Read the model definition and answer for the solid it produces. Units are mm, in the model's axes. Face numbers are marked on the shaded views. A direction names the side the tool comes from. Coordinates: 2 decimals unless noted, no trailing zeros. Write each loop counter-clockwise with the first axis right and the second up, starting at its lowest first coordinate (ties: lowest second). Pieces come first, ordered by that corner, then holes.
1) This flat-tipped pin is pushed along its axis until it touches: pin 1 Ø1.6 at (y, z) = (-2.66, -8.3) entering from +X. Where does it stop, or does it pass through?
2) Which of the six approach directions +Z, -Z, +X, -X, +Y, -Y give full straight-line access (tool end or side, diameter ignored) to the marked faces 5 and 6?
3) The part is cut by section A-A (y = -12). Determine the outline of the cut face in (x, z), then the cut area to 4 significant figures.
4) Determine the mould class of the marked faces 1, 2, 3 and 4 for opening direction X: +X half, -X half, draft (parallel to the pull), parting line (faces both ways), or undercut.
5) Find the intervals of material crossed by line 1 (X direction, y = -0.25, z = -15); line 2 (X direction, y = 3.5, z = 2.5); line 3 (Z direction, x = -4.5, y = -1), in increasing order.
6) The part is cut by section B-B (x = 20). Determine the outline of the cut face in (y, z), then the cut area to 3 significant figures.
from build123d import *

# Parameters (mm, degrees)
BOSS_EXTRUDE1_DEPTH = 5
SKETCH4_W           = 5
SKETCH4_H           = 30
BOSS_EXTRUDE4_DEPTH = 35
SKETCH5_R           = 3
CUT_EXTRUDE2_DEPTH  = 40
CUT_EXTRUDE3_DEPTH  = 10
SKETCH7_R           = 1
SKETCH7_R_2         = 1.000000019
CUT_EXTRUDE4_DEPTH  = 10
FILLET2_R           = 3
FILLET3_R           = 3
FILLET5_R           = 3
FILLET6_R           = 3
CUT_EXTRUDE5_DEPTH  = 5


with BuildPart() as part:
    # Sketch1 → Boss-Extrude1 (new body)
    with BuildSketch(Plane.XY):
        with BuildLine():
            Line((5, 0), (36.35, 0))
            Line((36.35, 0), (36.35, 15))
            Line((36.35, 15), (-36.35, 15))
            Line((-36.35, 15), (-36.35, 0))
            Line((-36.35, 0), (-5, 0))
            ThreePointArc((-5, 0), (0, 5), (5, 0))
        make_face()
        with BuildLine():
            ThreePointArc((-5, 0), (0, -5), (5, 0))
            Line((5, 0), (0, 0))
            Line((0, 0), (-5, 0))
        make_face()
        with BuildLine():
            Line((0, 0), (5, 0))
            ThreePointArc((5, 0), (0, 5), (-5, 0))
            Line((-5, 0), (0, 0))
        make_face()
        with BuildLine():
            Line((-36.35, -15), (36.35, -15))
            Line((36.35, -15), (36.35, 0))
            Line((36.35, 0), (5, 0))
            ThreePointArc((5, 0), (0, -5), (-5, 0))
            Line((-5, 0), (-36.35, 0))
            Line((-36.35, 0), (-36.35, -15))
        make_face()
    extrude(amount=BOSS_EXTRUDE1_DEPTH)

    # Sketch4 → Boss-Extrude4 (add)
    with BuildSketch(Plane(origin=(0, 0, 0), x_dir=(-1, 0, 0), z_dir=(0, 0, -1))):
        with Locations((-33.85, 0)):
            Rectangle(SKETCH4_W, SKETCH4_H)
    boss_extrude4 = extrude(amount=BOSS_EXTRUDE4_DEPTH)

    # Sketch5 → Cut-Extrude2 (cut)
    with BuildSketch(Plane(origin=(36.35, 0, 0), x_dir=(0, 0, -1), z_dir=(1, 0, 0))):
        with Locations(Location((20, 0, 0), (0, 0, 90))):
            Circle(SKETCH5_R)
    cut_extrude2 = extrude(amount=-CUT_EXTRUDE2_DEPTH, mode=Mode.SUBTRACT)

    # Sketch6 → Cut-Extrude3 (cut)
    with BuildSketch(Plane.ZY.offset(-31.35)):
        with BuildLine():
            ThreePointArc((-35, 0), (-30.606601718, 10.606601718), (-20, 15))
            Line((-20, 15), (-35, 15))
            Line((-35, 15), (-35, 0))
        make_face()
        with BuildLine():
            ThreePointArc((-20, -15), (-30.606601718, -10.606601718), (-35, 0))
            Line((-35, 0), (-35, -15))
            Line((-35, -15), (-20, -15))
        make_face()
    cut_extrude3 = extrude(amount=-CUT_EXTRUDE3_DEPTH, mode=Mode.SUBTRACT)

    # Sketch7 → Cut-Extrude4 (cut)
    with BuildSketch(Plane.ZY.offset(-31.35)):
        with Locations((-31.701517916, 2.659789178)):
            Circle(SKETCH7_R)
        with Locations((-17.340210822, 11.701517916)):
            Circle(SKETCH7_R)
        with Locations((-9.845022367, 6.393467704)):
            Circle(SKETCH7_R)
        with Locations((-30.154977622, -6.393467721)):
            Circle(SKETCH7_R_2)
        with Locations((-8.298482084, -2.659789178)):
            Circle(SKETCH7_R)
        with Locations((-26.393467704, 10.154977633)):
            Circle(SKETCH7_R)
        with Locations((-28.485281374, -8.485281374)):
            Circle(SKETCH7_R)
        with Locations((-20, -12)):
            Circle(SKETCH7_R)
    cut_extrude4 = extrude(amount=-CUT_EXTRUDE4_DEPTH, mode=Mode.SUBTRACT)

    # Fillet2
    fillet2_edges = [part.edges().sort_by_distance(p)[0] for p in [
        (36.35, 0, 5),
    ]]
    fillet(fillet2_edges, radius=FILLET2_R)

    # Fillet3
    fillet3_edges = [part.edges().sort_by_distance(p)[0] for p in [
        (31.35, 0, 0),
    ]]
    fillet(fillet3_edges, radius=FILLET3_R)

    # Mirror2: Boss-Extrude4, Cut-Extrude2, Cut-Extrude3, Cut-Extrude4 across plane
    add(boss_extrude4.mirror(Plane(origin=(0, 0, 0), x_dir=(0, 0, 1), z_dir=(1, 0, 0))))
    add(cut_extrude2.mirror(Plane(origin=(0, 0, 0), x_dir=(0, 0, 1), z_dir=(1, 0, 0))), mode=Mode.SUBTRACT)
    add(cut_extrude3.mirror(Plane(origin=(0, 0, 0), x_dir=(0, 0, 1), z_dir=(1, 0, 0))), mode=Mode.SUBTRACT)
    add(cut_extrude4.mirror(Plane(origin=(0, 0, 0), x_dir=(0, 0, 1), z_dir=(1, 0, 0))), mode=Mode.SUBTRACT)

    # Fillet5
    fillet5_edges = [part.edges().sort_by_distance(p)[0] for p in [
        (-36.35, 0, 5),
    ]]
    fillet(fillet5_edges, radius=FILLET5_R)

    # Fillet6
    fillet6_edges = [part.edges().sort_by_distance(p)[0] for p in [
        (-31.35, 0, 0),
    ]]
    fillet(fillet6_edges, radius=FILLET6_R)

    # Sketch9 → Cut-Extrude5 (cut)
    with BuildSketch(Plane.XY.offset(5)):
        with BuildLine():
            Line((3.977595735, 0.406889685), (3.197645987, 0.156889685))
            Line((3.197645987, 0.156889685), (3.197645987, -0.143110315))
            Line((3.197645987, -0.143110315), (3.977595735, -0.393110315))
            ThreePointArc((3.977595735, -0.393110315), (3.948399349, -0.618848175), (3.906409927, -0.842559818))
            Line((3.906409927, -0.842559818), (3.087379388, -0.83930622))
            Line((3.087379388, -0.83930622), (2.99467429, -1.124623174))
            Line((2.99467429, -1.124623174), (3.659196332, -1.603405031))
            ThreePointArc((3.659196332, -1.603405031), (3.561672083, -1.809072314), (3.452607071, -2.008859284))
            Line((3.452607071, -2.008859284), (2.674668157, -1.752670573))
            Line((2.674668157, -1.752670573), (2.498332581, -1.995375672))
            Line((2.498332581, -1.995375672), (2.982378869, -2.65607288))
            ThreePointArc((2.982378869, -2.65607288), (2.826073111, -2.82153744), (2.660608551, -2.977843197))
            Line((2.660608551, -2.977843197), (1.999911343, -2.493796909))
            Line((1.999911343, -2.493796909), (1.757206245, -2.670132485))
            Line((1.757206245, -2.670132485), (2.013394956, -3.448071399))
            ThreePointArc((2.013394956, -3.448071399), (1.813607986, -3.557136412), (1.607940702, -3.65466066))
            Line((1.607940702, -3.65466066), (1.129158846, -2.990138618))
            Line((1.129158846, -2.990138618), (0.843841891, -3.082843716))
            Line((0.843841891, -3.082843716), (0.847095489, -3.901874256))
            ThreePointArc((0.847095489, -3.901874256), (0.623383847, -3.943863677), (0.397645987, -3.973060063))
            Line((0.397645987, -3.973060063), (0.147645987, -3.193110315))
            Line((0.147645987, -3.193110315), (-0.152354013, -3.193110315))
            Line((-0.152354013, -3.193110315), (-0.402354013, -3.973060063))
            ThreePointArc((-0.402354013, -3.973060063), (-0.628091873, -3.943863677), (-0.851803516, -3.901874256))
            Line((-0.851803516, -3.901874256), (-0.848549918, -3.082843716))
            Line((-0.848549918, -3.082843716), (-1.133866873, -2.990138618))
            Line((-1.133866873, -2.990138618), (-1.612648729, -3.65466066))
            ThreePointArc((-1.612648729, -3.65466066), (-1.818316012, -3.557136412), (-2.018102983, -3.448071399))
            Line((-2.018102983, -3.448071399), (-1.761914272, -2.670132485))
            Line((-1.761914272, -2.670132485), (-2.00461937, -2.493796909))
            Line((-2.00461937, -2.493796909), (-2.665316578, -2.977843197))
            ThreePointArc((-2.665316578, -2.977843197), (-2.830781138, -2.82153744), (-2.987086896, -2.65607288))
            Line((-2.987086896, -2.65607288), (-2.503040607, -1.995375672))
            Line((-2.503040607, -1.995375672), (-2.679376183, -1.752670573))
            Line((-2.679376183, -1.752670573), (-3.457315097, -2.008859284))
            ThreePointArc((-3.457315097, -2.008859284), (-3.56638011, -1.809072314), (-3.663904358, -1.603405031))
            Line((-3.663904358, -1.603405031), (-2.999382316, -1.124623174))
            Line((-2.999382316, -1.124623174), (-3.092087415, -0.83930622))
            Line((-3.092087415, -0.83930622), (-3.911117954, -0.842559818))
            ThreePointArc((-3.911117954, -0.842559818), (-3.953107376, -0.618848175), (-3.982303762, -0.393110315))
            Line((-3.982303762, -0.393110315), (-3.202354013, -0.143110315))
            Line((-3.202354013, -0.143110315), (-3.202354013, 0.156889685))
            Line((-3.202354013, 0.156889685), (-3.982303762, 0.406889685))
            ThreePointArc((-3.982303762, 0.406889685), (-3.953107376, 0.632627545), (-3.911117954, 0.856339187))
            Line((-3.911117954, 0.856339187), (-3.092087415, 0.85308559))
            Line((-3.092087415, 0.85308559), (-2.999382316, 1.138402544))
            Line((-2.999382316, 1.138402544), (-3.663904358, 1.617184401))
            ThreePointArc((-3.663904358, 1.617184401), (-3.56638011, 1.822851684), (-3.457315097, 2.022638654))
            Line((-3.457315097, 2.022638654), (-2.679376183, 1.766449943))
            Line((-2.679376183, 1.766449943), (-2.503040607, 2.009155041))
            Line((-2.503040607, 2.009155041), (-2.987086896, 2.66985225))
            ThreePointArc((-2.987086896, 2.66985225), (-2.830781138, 2.83531681), (-2.665316578, 2.991622567))
            Line((-2.665316578, 2.991622567), (-2.00461937, 2.507576279))
            Line((-2.00461937, 2.507576279), (-1.761914272, 2.683911855))
            Line((-1.761914272, 2.683911855), (-2.018102983, 3.461850769))
            ThreePointArc((-2.018102983, 3.461850769), (-1.818316012, 3.570915782), (-1.612648729, 3.66844003))
            Line((-1.612648729, 3.66844003), (-1.133866873, 3.003917988))
            Line((-1.133866873, 3.003917988), (-0.848549918, 3.096623086))
            Line((-0.848549918, 3.096623086), (-0.851803516, 3.915653625))
            ThreePointArc((-0.851803516, 3.915653625), (-0.628091873, 3.957643047), (-0.402354013, 3.986839433))
            Line((-0.402354013, 3.986839433), (-0.152354013, 3.206889685))
            Line((-0.152354013, 3.206889685), (0.147645987, 3.206889685))
            Line((0.147645987, 3.206889685), (0.397645987, 3.986839433))
            ThreePointArc((0.397645987, 3.986839433), (0.623383847, 3.957643047), (0.847095489, 3.915653625))
            Line((0.847095489, 3.915653625), (0.843841891, 3.096623086))
            Line((0.843841891, 3.096623086), (1.129158846, 3.003917988))
            Line((1.129158846, 3.003917988), (1.607940702, 3.66844003))
            ThreePointArc((1.607940702, 3.66844003), (1.813607986, 3.570915782), (2.013394956, 3.461850769))
            Line((2.013394956, 3.461850769), (1.757206245, 2.683911855))
            Line((1.757206245, 2.683911855), (1.999911343, 2.507576279))
            Line((1.999911343, 2.507576279), (2.660608551, 2.991622567))
            ThreePointArc((2.660608551, 2.991622567), (2.826073111, 2.83531681), (2.982378869, 2.66985225))
            Line((2.982378869, 2.66985225), (2.498332581, 2.009155041))
            Line((2.498332581, 2.009155041), (2.674668157, 1.766449943))
            Line((2.674668157, 1.766449943), (3.452607071, 2.022638654))
            ThreePointArc((3.452607071, 2.022638654), (3.561672083, 1.822851684), (3.659196332, 1.617184401))
            Line((3.659196332, 1.617184401), (2.99467429, 1.138402544))
            Line((2.99467429, 1.138402544), (3.087379388, 0.85308559))
            Line((3.087379388, 0.85308559), (3.906409927, 0.856339187))
            ThreePointArc((3.906409927, 0.856339187), (3.948399349, 0.632627545), (3.977595735, 0.406889685))
        make_face()
    extrude(amount=-CUT_EXTRUDE5_DEPTH, mode=Mode.SUBTRACT)


solid = part.part
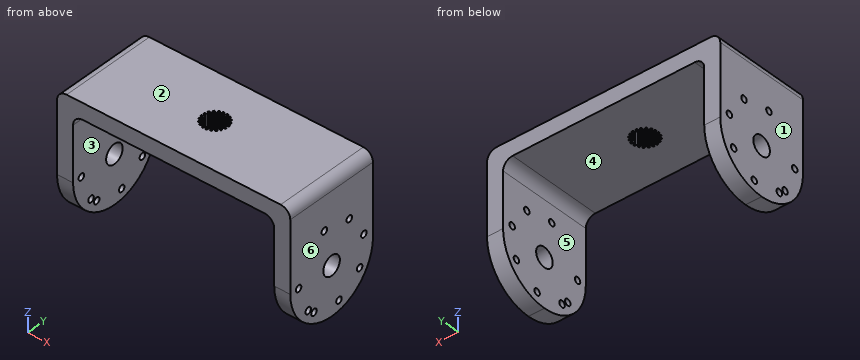
Reported:
1. pin 1: passes through
2. face 5: -Z, +Y, -Y
2. face 6: +Z, -Z, +X, +Y, -Y
3. outline: (-36.35, -29) - (-31.35, -29) - (-31.35, -21) - (-36.35, -21) - close; (-36.35, -19) - (-31.35, -19) - (-31.35, -3) arc R3 cw to (-28.35, 0) - (28.35, 0) arc R3 cw to (31.35, -3) - (31.35, -19) - (36.35, -19) - (36.35, 2) arc R3 ccw to (33.35, 5) - (-33.35, 5) arc R3 ccw to (-36.35, 2) - close; (31.35, -29) - (36.35, -29) - (36.35, -21) - (31.35, -21) - close
3. area: 633.5 mm2
4. face 1: -X half
4. face 2: draft
4. face 3: undercut
4. face 4: undercut
5. line 1: x = -36.35 to -31.35, 31.35 to 36.35
5. line 2: x = -36.31 to -1.95, -1.49 to -0.85, -0.25 to 0.24, 0.85 to 1.49, 1.95 to 36.31
5. line 3: z = 0 to 5
6. outline: (-15, 0) - (15, 0) - (15, 5) - (-15, 5) - close
6. area: 150 mm2
